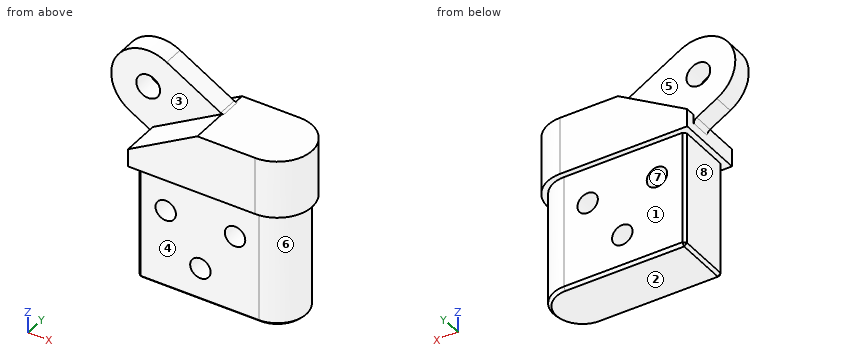
```python
from build123d import *

# Parameters (mm, degrees)
F1_DEPTH = 15.875
F3_DEPTH = 31.75
F4_SIZE2 = 10.9985226281
F4_SIZE  = 19.05
F6_START = -2.794
F6_DEPTH = 5.715
F8_D     = 6.5278
F9_SIZE  = 0.762
F11_D    = 5.6134
F12_R    = 1.5875


with BuildPart() as f1:
    # F0 (on Top) → F1 (new body)
    with BuildSketch(Plane.XY):
        with BuildLine():
            Line((0, 9.525), (-34.925, 9.525))
            Line((-34.925, 9.525), (-34.925, -9.525))
            Line((-34.925, -9.525), (0, -9.525))
            ThreePointArc((0, -9.525), (9.525, 0), (0, 9.525))
        make_face()
    extrude(amount=-F1_DEPTH)

    # F2 (on face) → F3 (join)
    with BuildSketch(Plane(origin=(0, 0, -15.875), x_dir=(1, 0, 0), z_dir=(0, 0, -1))):
        with BuildLine():
            Line((0, 7.9375), (-33.3375, 7.9375))
            Line((-33.3375, 7.9375), (-33.3375, -7.9375))
            Line((-33.3375, -7.9375), (0, -7.9375))
            ThreePointArc((0, -7.9375), (7.9375, 0), (0, 7.9375))
        make_face()
    extrude(amount=F3_DEPTH)

    # F4
    f4_edges = [f1.edges().sort_by_distance(p)[0] for p in [
        (-34.925, 0, 0),
    ]]
    f4_side = f1.faces().sort_by_distance((-13.668751, 0, 0))[0]
    chamfer(f4_edges, length=F4_SIZE, length2=F4_SIZE2, reference=f4_side)

    # F5 (on face) → F6 (join)
    with BuildSketch(Plane(origin=(0, 9.525, 0), x_dir=(-1, 0, 0), z_dir=(0, 1, 0)).offset(F6_START)):
        with BuildLine():
            Line((34.925, -12.4649923118), (41.275, -8.7988181024))
            ThreePointArc((41.275, -8.7988181024), (44.9938181024, 5.08), (31.115, 8.7988181024))
            Line((31.115, 8.7988181024), (15.875, 0))
            Line((15.875, 0), (34.925, -10.9985226281))
            Line((34.925, -10.9985226281), (34.925, -12.4649923118))
        make_face()
    extrude(amount=-F6_DEPTH)

    # F8 (through all)
    with Locations(Plane(origin=(0, 6.731, 0), x_dir=(-1, 0, 0), z_dir=(0, 1, 0))):
        with Locations((36.195, 0)):
            Hole(F8_D / 2)

    # F9
    f9_edges = [f1.edges().sort_by_distance(p)[0] for p in [
        (-16.66875, -7.9375, -47.625),
        (-33.3375, 0, -47.625),
        (-33.3375, -7.9375, -31.75),
        (-33.3375, 7.9375, -31.75),
        (7.9375, 0, -47.625),
        (-16.66875, 7.9375, -47.625),
    ]]
    chamfer(f9_edges, length=F9_SIZE)

    # F11 (through all)
    with Locations(Plane(origin=(0, 7.9375, 0), x_dir=(-1, 0, 0), z_dir=(0, 1, 0))):
        with Locations((25.5905, -25.7175), (6.5405, -25.7175), (16.0655, -38.4175)):
            Hole(F11_D / 2)

    # F12
    f12_edges = [f1.edges().sort_by_distance(p)[0] for p in [
        (-15.875, 3.8735, 0),
        (-34.925, 3.8735, -12.464992),
    ]]
    fillet(f12_edges, radius=F12_R)


solid = f1.part
```
Verification items for the finished model (mm, model axes). Face numbers are marked on the shaded views. A direction names the side the tool comes from. Give positions to 0.01 mm unless a question says otherwise; leave off trailing zeros. Loops run counter-clockwise (first coordinate to the right, second up) from the corner with the lowest first, then second, coordinate; pieces in that order, holes last.
1. Section check A-A, the plane x = -26.5. Enter the section's corners in (y, z) (1 decimal).
2. Mould release check, pull along X, two halves, no side actions. Record for the marked faces 6, 7 and 8: released by +X, released by -X, zero draft, split by the parting line, or undercut.
3. Set-up check for the marked faces 1, 2, 3, 4 and 5: record each of +Z, -Z, +X, -X, +Y, -Y from which the full face is reachable in a straight line by a thin tool's end or side.
4. Go/stop test with flat-tipped pins: pin 1 Ø25 at (x, z) = (-11, -33.5) entering from -Y; pin 2 Ø3 at (y, z) = (-0.5, -21.5) entering from -X; pin 3 Ø10 at (x, y) = (-12, -6) entering from +Z. Record where each tip stops, or that it passes through.
5. Section check B-B, the plane z = -37.5. Enter the section's corners in (x, y) (1 decimal).
6. Section check C-C, the plane y = 0. Enter the section's corners in (x, z) (1 decimal), then the cut area to 3 significant figures.
7. Thickness scan on line 1 (X direction, y = -5.5, z = -27); line 2 (X direction, y = 4.5, z = -24.5); line 3 (Y direction, x = -4, z = -16.5). Record the ranges inside material, lowest first.
8. Section check D-D, the plane z = -20.5. Enter the section's corners in (x, y) (1 decimal), then the cut area to 3 significant figures.
Geometry says:
1. outline: (-9.5, -15.9) - (-7.9, -15.9) - (-7.9, -23.1) - (7.9, -23.1) - (7.9, -15.9) - (9.5, -15.9) - (9.5, -6.1) - (6.7, -6.1) - (6.7, 6.1) - (1, 6.1) - (1, -6.1) - (-9.5, -6.1) - close; (-7.9, -46.9) - (-7.2, -47.6) - (7.2, -47.6) - (7.9, -46.9) - (7.9, -28.4) - (-7.9, -28.4) - close
2. face 6: released by +X
2. face 7: undercut
2. face 8: released by -X
3. face 1: -Z, +X, -X, +Y
3. face 2: -Z, +X, -X, +Y, -Y
3. face 3: +Z, -X, -Y
3. face 4: -Z, +X, -X, -Y
3. face 5: +Z, -X, +Y
4. pin 1: stops at y = -7.94
4. pin 2: stops at x = -33.34
4. pin 3: stops at z = 0
5. outline: (-33.3, -7.2) - (-32.6, -7.9) - (-18.7, -7.9) - (-18.7, 7.9) - (-32.6, 7.9) - (-33.3, 7.2) - close; (-13.4, -7.9) - (0, -7.9) arc R7.9 ccw to (0, 7.9) - (-13.4, 7.9) - close
6. outline: (-34.9, -15.9) - (-33.3, -15.9) - (-33.3, -46.9) - (-32.6, -47.6) - (7.2, -47.6) - (7.9, -46.9) - (7.9, -15.9) - (9.5, -15.9) - (9.5, 0) - (-15.9, 0) - (-34.9, -11) - close; hole circle Ø5.6 at (-25.6, -25.7); hole circle Ø5.6 at (-16.1, -38.4); hole circle Ø5.6 at (-6.5, -25.7)
6. area: 1,840 mm2
7. line 1: x = -33.34 to -28.09, -23.09 to -9.04, -4.04 to 5.72
7. line 2: x = -33.34 to -28.12, -23.06 to -9.07, -4.01 to 6.54
7. line 3: y = -7.94 to 7.94
8. outline: (-33.3, -7.2) - (-32.6, -7.9) - (0, -7.9) arc R7.9 ccw to (0, 7.9) - (-32.6, 7.9) - (-33.3, 7.2) - close
8. area: 628 mm2
